Input: part model. Units: mm. Frame: model coordinates. Face numbers are marked on the shaded views. A direction names the side the tool comes from. Coordinates: 2 decimals unless noted, no trailing zeros. Write each loop counter-clockwise with the first axis right and the second up, starting at its lowest first coordinate (ties: lowest second). Pieces come first, ordered by that corner, then holes. Notation, with made-up numbers: (-26.75, 68.25) - (8.25, 68.25) arc R25 cw to (8.25, 95.25) - close; hole circle Ø5 at (-0.75, 53.25). An arc over 180 degrees is marked (long way). Use CSV: the item, a comma, the result in double quotes.
```python
from build123d import *

# Parameters (mm, degrees)
SKETCH2_R                          = 2.5
CUT_EXTRUDE1_DEPTH                 = 10
SKETCH3_R                          = 1.5
CUT_EXTRUDE2_DEPTH                 = 8
SKETCH4_R                          = 1.5
CUT_EXTRUDE3_DEPTH                 = 4
SKETCH5_R                          = 1.5
CUT_EXTRUDE4_DEPTH                 = 4
CUT_EXTRUDE7_DEPTH                 = 10
CUT_EXTRUDE7_DEPTH_BACK            = 10
SKETCH6_R                          = 2.5
BOSS_EXTRUDE5_DEPTH                = 5
BOSS_EXTRUDE5_DEPTH_BACK           = 5
F_5_0_5_DIAMETER_HOLE1_D           = 5
F_5_0_5_DIAMETER_HOLE1_ON_FACE_2_D = 5


with BuildPart() as part:
    # Sketch1 → Revolve2 (revolve)
    with BuildSketch(Plane.XY, mode=Mode.PRIVATE) as revolve2_sk:
        Polygon((5, 7.28), (5, 0), (30, 0), (30, 25), (25, 25), (25, 5), (12.5, 5), (12.5, 23.98), (5, 23.98), (5, 11.48), (7, 11.48), (7, 7.28), align=None)
    revolve(revolve2_sk.sketch.rotate(Axis((0, 23.98, 0), (0, -1, 0)), 180), axis=Axis((0, 23.98, 0), (0, -1, 0)))

    # Sketch2 → Cut-Extrude1 (cut)
    with BuildSketch(Plane.XZ):
        with Locations((0, -19)):
            Circle(SKETCH2_R)
    extrude(amount=-CUT_EXTRUDE1_DEPTH, mode=Mode.SUBTRACT)

    # Sketch3 → Cut-Extrude2 (cut)
    with BuildSketch(Plane(origin=(0, 23.98, 0), x_dir=(1, 0, 0), z_dir=(0, 1, 0))):
        with Locations(Location((-8.5, 0, 0), (0, 0, 180))):
            Circle(SKETCH3_R)
        with Locations(Location((0, 8.5, 0), (0, 0, 180))):
            Circle(SKETCH3_R)
    extrude(amount=-CUT_EXTRUDE2_DEPTH, mode=Mode.SUBTRACT)

    # Sketch4 → Cut-Extrude3 (cut)
    with BuildSketch(Plane.XY.offset(-12.5)):
        with Locations(Location((0, 17.5, 0), (0, 0, 180))):
            Circle(SKETCH4_R)
    extrude(amount=CUT_EXTRUDE3_DEPTH, mode=Mode.SUBTRACT)

    # Sketch5 → Cut-Extrude4 (cut)
    with BuildSketch(Plane(origin=(-12.5, 0, 0), x_dir=(0, 0, -1), z_dir=(1, 0, 0))):
        with Locations(Location((0, 17.5, 0), (0, 0, 270))):
            Circle(SKETCH5_R)
    extrude(amount=CUT_EXTRUDE4_DEPTH, mode=Mode.SUBTRACT)

    # Sketch6 → Cut-Extrude7 (cut, two sides: drawn at the far end of the back side and taken through both)
    with BuildSketch(Plane(origin=(-30, 0, 0), x_dir=(0, 0, -1), z_dir=(1, 0, 0)).offset(-CUT_EXTRUDE7_DEPTH_BACK)):
        with Locations(Location((0, 17.5, 0), (0, 0, 90))):
            Circle(SKETCH6_R)
    extrude(amount=CUT_EXTRUDE7_DEPTH + CUT_EXTRUDE7_DEPTH_BACK, mode=Mode.SUBTRACT)

    # Sketch7 → Boss-Extrude5 (add, two sides: drawn at the far end of the back side and taken through both)
    with BuildSketch(Plane.XY.offset(-BOSS_EXTRUDE5_DEPTH_BACK)):
        with BuildLine():
            Line((-32, 0), (-30, 0))
            Line((-30, 0), (-15, 0))
            Line((-15, 0), (-15, -9.5))
            ThreePointArc((-15, -9.5), (-15.878679656, -11.621320344), (-18, -12.5))
            Line((-18, -12.5), (-32, -12.5))
            ThreePointArc((-32, -12.5), (-34.121320344, -11.621320344), (-35, -9.5))
            Line((-35, -9.5), (-35, -3))
            ThreePointArc((-35, -3), (-34.121320344, -0.878679656), (-32, 0))
        make_face()
    extrude(amount=BOSS_EXTRUDE5_DEPTH + BOSS_EXTRUDE5_DEPTH_BACK)

    # 5.0 _5_ Diameter Hole1 (through all)
    with Locations(Plane(origin=(-25, -8, -5), x_dir=(-1, 0, 0), z_dir=(0, 0, -1))):
        with Locations((0, 0)):
            Hole(F_5_0_5_DIAMETER_HOLE1_D / 2)

    # 5.0 _5_ Diameter Hole1 on face 2 (through all)
    with Locations(Plane(origin=(-19.5551144, -17.55502899, 0), x_dir=(-1, 0, 0), z_dir=(0, 0, -1))):
        with Locations((0, 0)):
            Hole(F_5_0_5_DIAMETER_HOLE1_ON_FACE_2_D / 2)


solid = part.part
```
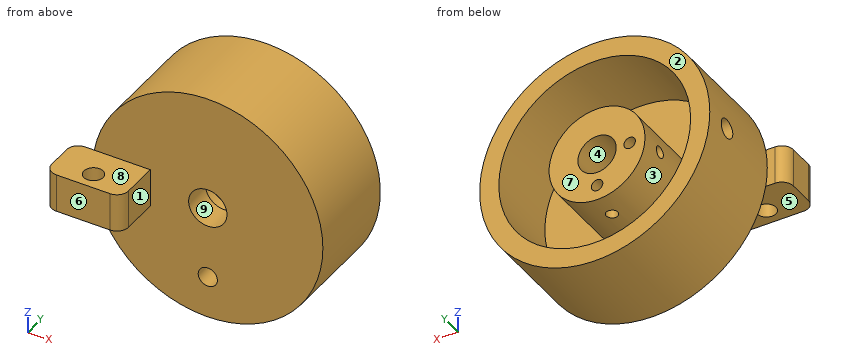
(1) Cut plane C-C on y = 8.5. Return loops of the section in (x, z), and give its area (3 significant figures).
Check values:
outline,"circle Ø60 at (0, 0); circle Ø25 at (0, 0); hole circle Ø50 at (0, 0); hole circle Ø14 at (0, 0)"
area,"1,200 mm^2"
(2) Draft query along Z for the marked faces 6, 7, 8 and 9. Return one class per face: pulls with the +Z half, pulls with the -Z half, needs draft (parallel to the pull), parting line crosses it, or undercut.
Check values:
face 6,"needs draft"
face 7,"undercut"
face 8,"pulls with the +Z half"
face 9,"undercut"
(3) Cut plane B-B on z = -19. Return loops of the section in (x, y), and give its area (3 significant figures).
Check values:
outline,"(-23.22, 0) - (-2.5, 0) - (-2.5, 5) - (-16.25, 5) - (-16.25, 25) - (-23.22, 25) - close; (2.5, 0) - (23.22, 0) - (23.22, 25) - (16.25, 25) - (16.25, 5) - (2.5, 5) - close"
area,"486 mm^2"
(4) Pin query (flat end, axial travel): pin 1 Ø6 at (y, z) = (5, -0.5) entering from -X; pin 2 Ø3.5 at (x, z) = (-8.5, 0) entering from +Y; pin 3 Ø2 at (x, z) = (0, 24) entering from -Y. Return the tip coordinate at first contact, or that it passes through.
Check values:
pin 1,"x = -30"
pin 2,"y = 23.98"
pin 3,"y = 0"
(5) Cut plane A-A on y = -8. Return loops of the section in (x, z).
Check values:
outline,"(-35, -5) - (-27.5, -5) - (-27.5, 5) - (-35, 5) - close; (-22.5, -5) - (-15, -5) - (-15, 5) - (-22.5, 5) - close"
(6) Cut plane D-D on z = 0. State how many separate pieces and enclosed holes the cut face has, and give its area (3 significant figures).
Check values:
separate pieces,"4"
enclosed holes,"1"
area,"886 mm^2"
(7) Reachability of the marked faces 1, 2, 3, 4 and 5 from +Z, -Z, +X, -X, +Y, -Y: full face, straight path, thin tool, end or side. Return the list, or none.
Check values:
face 1,"+Z, -Z, +X, -Y"
face 2,"+Z, -Z, +X, -X, +Y"
face 3,"+Y"
face 4,"+Y, -Y"
face 5,"-Z, +X, -X, -Y"
(8) Ray query, probe 1 along Z at (x, y) = (0, 12); probe 2 along Z at (x, y) = (0, 20.75); probe 3 along Z at (x, y) = (0, 18.5). Return the intervals inside material, ascending. Write a range as from..to.
Check values:
probe 1,"-30..-25, -12.5..-5, 5..12.5, 25..30"
probe 2,"-30..-25, -12.5..-10, -7..-5, 5..12.5, 25..30"
probe 3,"-30..-25, -7..-5, 5..12.5, 25..30"
